Autodesk Inventor part; units mm, degrees
ref_plane "YZ Plane" through (0, 0, 0) normal (1, 0, 0) x (0, 1, 0)
ref_plane "XZ Plane" through (0, 0, 0) normal (0, 1, 0) x (-1, 0, 0)
ref_plane "XY Plane" through (0, 0, 0) normal (0, 0, 1) x (1, 0, 0)
sketch "Sketch4" plane through (0, 0, 0) normal (0, 1, 0) x (-1, 0, 0)
  line L0 (0, 0) -> (26.67, 0)
  line L1 (26.67, 0) -> (26.67, 20.066)
  line L2 (26.67, 20.066) -> (0, 20.066)
  line L3 (0, 20.066) -> (0, 0)
  dimension "d20" = 20.066
  dimension "d21" = 26.67
extrude "Extrusion4" add sketch "Sketch4" along normal blind 1.651
sketch "Sketch5" plane through (0, 1.651, 0) normal (0, 1, 0) x (1, 0, 0)
  line L0 (-26.67, -20.066) -> (0, -20.066)
  line L1 (-25.4, -20.066) -> (-1.27, -20.066)
  line L2 (-1.27, -20.066) -> (-1.27, 0)
  line L3 (-1.27, 0) -> (-25.4, 0)
  line L4 (-25.4, 0) -> (-25.4, -20.066)
  line L5 (-26.67, 0) -> (-26.67, -20.066)
  line L6 (0, 0) -> (-26.67, 0)
  line L7 (0, -20.066) -> (0, 0)
  point P0 (-1.27, -20.066)
  dimension "d24" = 1.27
  dimension "d25" = 0
  dimension "d26" = 1.27
extrude "Extrusion5" add sketch "Sketch5" along normal blind 1.524 contours L4 L3 L2 L0
sketch "Sketch8" plane through (-26.67, 0, 20.066) normal (0, 0, 1) x (1, 0, 0)
  line L0 (3.175, 1.651) -> (23.495, 1.651)
  line L1 (23.495, 1.651) -> (23.495, 0)
  line L2 (23.495, 0) -> (3.175, 0)
  line L3 (3.175, 0) -> (3.175, 1.651)
  line L4 (0, 0) -> (26.67, 0)
  line L5 (26.67, 0) -> (26.67, 1.651)
  line L6 (0, 0) -> (0, 1.651)
  dimension "d42" = 20.32
  dimension "d43" = 1.651
  dimension "d44" = 0
  dimension "d45" = 26.67
  dimension "d46" = 3.175
extrude "Extrusion8" add sketch "Sketch8" along normal blind 5.08
sketch "Sketch9" plane through (-23.495, 1.651, 20.066) normal (0, 1, 0) x (1, 0, 0)
  line L0 (0, 0) -> (0, -5.08)
  line L1 (20.32, -2.54) -> (0, -2.54)
  line L2 (0, 0) -> (20.32, 0)
  line L3 (20.32, 0) -> (20.32, -2.54)
  line L4 (20.32, -2.54) -> (0, -2.54)
  line L5 (0, -2.54) -> (0, 0)
  point P0 (23.495, 20.066)
extrude "Extrusion9" add sketch "Sketch9" along normal blind 1.524
equation "\"d26\" = d24"
equation "\"d46\" = -0.5 * d42 + 0.5 * d45"
properties part number "_3DPrint"
Read the model definition and answer for the solid it produces. Units are mm, in the model's axes. A direction names the side the tool comes from. Coordinates: 2 decimals unless noted, no trailing zeros. Write each loop counter-clockwise with the first axis right and the second up, starting at its lowest first coordinate (ties: lowest second). Pieces come first, ordered by that corner, then holes. Notation, with made-up numbers: (17, -10) - (67, -10) arc R10 cw to (67, -2) - close; hole circle Ø1 at (18, 48). An arc over 180 degrees is marked (long way). Answer as a JSON object with one key per item and string values. Group by question number.
1. A cutting plane is placed at A-A (y = 2.4). Determine the outline of the cut face in (x, z) (3 decimals).
2. A cutting plane is placed at B-B (z = 19). Determine the outline of the cut face in (x, y) (3 decimals).
3. Which of the six approach directions +Z, -Z, +X, -X, +Y, -Y give full straight-line access (tool end or side, diameter ignored) to faces 1 (the flat face through (-1.27, 2, 10)), 2 (the flat face through (-2, 1, 20.066)), 3 (the flat face through (-25.4, 2, 10)), 4 (the flat face through (-13, 1.651, 24)), 5 (the flat face through (-23.495, 1, 22))?
4. A cutting plane is placed at C-C (x = -19). Determine the outline of the cut face in (y, z) (3 decimals), plus the area to 3 significant figures.
5. Consider L1, parallel to X at y = 2.55, z = 4; L2, parallel to Z at x = -1.25, y = 1.45; L3, parallel to Z at x = -11, y = 2.5. Determine where each line is inside the solid, lowest interval first. Write a range as [from, to].
6. Each of these flat-tipped pins is pushed along its axis until it touches: P1, Ø1.2, axis at x = -16, y = 2.5, coming from the +Z side; P2, Ø0.8, axis at y = 3, z = 5, coming from the +X side; P3, Ø1.6, axis at x = -25.5, y = 1.5, coming from the +Z side. Where does it stop, or does it pass through?
Worked out:
{
 "1": {"outline": "(-25.4, 0) - (-1.27, 0) - (-1.27, 20.066) - (-3.175, 20.066) - (-3.175, 22.606) - (-23.495, 22.606) - (-23.495, 20.066) - (-25.4, 20.066) - close"},
 "2": {"outline": "(-26.67, 0) - (0, 0) - (0, 1.651) - (-1.27, 1.651) - (-1.27, 3.175) - (-25.4, 3.175) - (-25.4, 1.651) - (-26.67, 1.651) - close"},
 "3": {"face 1": "+Z, -Z, +X, +Y", "face 2": "+Z, +X, +Y, -Y", "face 3": "+Z, -Z, -X, +Y", "face 4": "+Z, +X, -X, +Y", "face 5": "+Z, -X, +Y, -Y"},
 "4": {"outline": "(0, 0) - (3.175, 0) - (3.175, 22.606) - (1.651, 22.606) - (1.651, 25.146) - (0, 25.146) - close", "area": "76.0 mm²"},
 "5": {"L1": "x = [-25.4, -1.27]", "L2": "z = [0, 20.07]", "L3": "z = [0, 22.61]"},
 "6": {"P1": "stops at z = 22.61", "P2": "stops at x = -1.27", "P3": "stops at z = 20.07"}
}
